Check sheet for the modelled part. Datum: model origin and axes. Units: mm. A direction names the side the tool comes from. Round coordinates to 2 decimals unless told otherwise and drop trailing zeros. Write each loop counter-clockwise with the first axis right and the second up, starting at its lowest first coordinate (ties: lowest second). Pieces come first, ordered by that corner, then holes.
Item 1: Go/stop test with flat-tipped pins: pin 1 Ø17.5 at (y, z) = (200, 134) entering from +X; pin 2 Ø3 at (x, z) = (218, 129.5) entering from -Y; pin 3 Ø2 at (y, z) = (195.5, 125) entering from +X; pin 4 Ø14.5 at (x, z) = (200, 130) entering from -Y. Record where each tip stops, or that it passes through.
Item 2: Cross-section at A-A on z = 140.5. Enter the section's corners in (x, y), plus the area to 3 significant figures.
Item 3: Tool access check on faces 1 (the cylindrical face through (217, 200, 138)), 2 (the cylindrical face through (200, 217, 138)), 3 (the flat face through (200, 200, 150)). Record the directions out of +Z, -Z, +X, -X, +Y, -Y that give a thin tool (end or side, any length) a straight path to the whole face; none if there is none.
Item 4: Material ranges on line 1 (Z direction, x = 215, y = 200); line 2 (Y direction, x = 214, z = 130); line 3 (X direction, y = 220, z = 130), recorded low to high.
Item 5: Release check for a two-part mould opening along X. For faces 4 (the flat face through (200, 200, 110)), 5 (the flat face through (210, 200, 130)), 6 (the cylindrical face through (194.581, 175.594, 130.266)), 7 (the flat face through (200, 210, 130)) record: +X half, -X half, draft (parallel to the pull), parting line (faces both ways), or undercut.
from build123d import *

# Parameters (mm, degrees)
SKETCH20_R          = 25
BOSS_EXTRUDE6_DEPTH = 40
SKETCH21_R          = 8
CUT_EXTRUDE2_DEPTH  = 26
CIRPATTERN1_COUNT   = 2
CIRPATTERN1_ANGLE   = 90
FILLET5_R           = 1


with BuildPart() as part:
    # Sketch20 → Boss-Extrude6 (new body)
    with BuildSketch(Plane.XY.offset(150)):
        with Locations((200, 200)):
            Circle(SKETCH20_R)
    extrude(amount=-BOSS_EXTRUDE6_DEPTH)

    # Sketch21 → Cut-Extrude2 (cut)
    with BuildSketch(Plane(origin=(0, 210, 0), x_dir=(1, 0, 0), z_dir=(0, 1, 0))):
        with Locations(Location((200, -130, 0), (0, 0, 90))):
            Circle(SKETCH21_R)
    cut_extrude2 = extrude(amount=CUT_EXTRUDE2_DEPTH, mode=Mode.SUBTRACT)

    # CirPattern1: Cut-Extrude2 ×2 about axis
    cirpattern1_axis = Axis((200, 200, 110), (0, 0, -1))
    for i in range(1, CIRPATTERN1_COUNT):
        add(cut_extrude2.rotate(cirpattern1_axis, i * CIRPATTERN1_ANGLE / (CIRPATTERN1_COUNT - 1)), mode=Mode.SUBTRACT)

    # Fillet5
    fillet5_edges = [part.edges().sort_by_distance(p)[0] for p in [
        (223.685438565, 208, 130),
        (175, 200, 150),
        (175, 200, 110),
        (200, 224.999999999, 138.000000001),
    ]]
    fillet(fillet5_edges, radius=FILLET5_R)


solid = part.part
Response values:
1. pin 1: stops at x = 225
1. pin 2: stops at y = 181.22
1. pin 3: stops at x = 210
1. pin 4: stops at y = 175
2. outline: circle Ø50 at (200, 200)
2. area: 1,960 mm2
3. face 1: +X
3. face 2: +Y
3. face 3: +Z, +X, -X, +Y, -Y
4. line 1: z = 110 to 122, 138 to 150
4. line 2: y = 179.29 to 192, 208 to 220.71
4. line 3: x = 185 to 192, 208 to 215
5. face 4: draft
5. face 5: +X half
5. face 6: parting line
5. face 7: undercut
